Model file for the job. Use its own axes, mm. Face numbers are marked on the shaded views. A direction names the side the tool comes from. Give positions to 0.01 mm unless a question says otherwise; leave off trailing zeros. Loops run counter-clockwise (first coordinate to the right, second up) from the corner with the lowest first, then second, coordinate; pieces in that order, holes last. Notation, with made-up numbers: M -3,25 L 52,25 A26 cw 52,39 Z; hole C 27,-28.75 d2. An arc over 180 degrees is marked long. Answer in a Markdown table with one row per item.
```python
from build123d import *

# Parameters (mm, degrees)
SKETCH1_R                = 5
BOSS_EXTRUDE2_DEPTH      = 26
SKETCH9_R                = 11.5
CUT_EXTRUDE7_DEPTH       = 26
CUT_EXTRUDE8_DEPTH       = 57
BOSS_EXTRUDE5_DEPTH      = 35
BOSS_EXTRUDE5_DEPTH_BACK = 10


with BuildPart() as part:
    # Sketch1 → Boss-Extrude2 (new body)
    with BuildSketch(Plane.XY):
        with BuildLine():
            Line((-13.871543988, -187.456565175), (-0.750718318, -9.931237526))
            Line((-0.750718318, -9.931237526), (-9.971378105, 32.063387678))
            Line((-9.971378105, 32.063387678), (-9.97665526, 32.075234554))
            Line((-9.97665526, 32.075234554), (-9.977087782, 32.075348974))
            Line((-9.977087782, 32.075348974), (-9.978230603, 32.075651298))
            Line((-9.978230603, 32.075651298), (-9.977087779, 32.075655544))
            ThreePointArc((-9.977087779, 32.075655544), (-24.981119404, 47.075655002), (-39.977085612, 32.067592296))
            Line((-39.977085612, 32.067592296), (-40.143970803, 31.267359869))
            Line((-40.143970803, 31.267359869), (-33.520138903, -191.065133081))
            ThreePointArc((-33.520138903, -191.065133081), (-31.855635546, -197.51068285), (-27.565830072, -202.601188939))
            Line((-27.565830072, -202.601188939), (-6.826859709, -218.262215052))
            Line((-6.826859709, -218.262215052), (-2.296825809, -203.937706242))
            Line((-2.296825809, -203.937706242), (-10.96981355, -195.264718501))
            ThreePointArc((-10.96981355, -195.264718501), (-13.272387355, -191.677160819), (-13.871543988, -187.456565175))
        make_face()
        with Locations((-18.750718318, -9.924344456)):
            Circle(SKETCH1_R, mode=Mode.SUBTRACT)
    extrude(amount=BOSS_EXTRUDE2_DEPTH)

    # Sketch9 → Cut-Extrude7 (cut)
    with BuildSketch(Plane.XY):
        with Locations((-24.977087779, 32.075655544)):
            Circle(SKETCH9_R)
    extrude(amount=CUT_EXTRUDE7_DEPTH, mode=Mode.SUBTRACT)

    # Sketch10 → Cut-Extrude8 (cut)
    with BuildSketch(Plane.XY):
        with BuildLine():
            Line((-29.654511548, -21.002260091), (-10.602832717, -21.002260091))
            ThreePointArc((-10.602832717, -21.002260091), (-6.952180176, -22.585721488), (-5.613794584, -26.333165681))
            Line((-5.613794584, -26.333165681), (-9.366001824, -82.90490561))
            ThreePointArc((-9.366001824, -82.90490561), (-10.938501354, -86.224652561), (-14.355039957, -87.574000019))
            Line((-14.355039957, -87.574000019), (-27.922723591, -87.574000019))
            ThreePointArc((-27.922723591, -87.574000019), (-31.403747307, -86.163216354), (-32.920382463, -82.726989577))
            Line((-32.920382463, -82.726989577), (-34.65217042, -26.155249648))
            ThreePointArc((-34.65217042, -26.155249648), (-33.243727882, -22.521236375), (-29.654511548, -21.002260091))
        make_face()
        with BuildLine():
            Line((-14.784895538, -91.270958439), (-27.832276958, -91.270958439))
            ThreePointArc((-27.832276958, -91.270958439), (-31.398552804, -92.766436134), (-32.831514258, -96.358287804))
            Line((-32.831514258, -96.358287804), (-31.399590979, -178.329847134))
            ThreePointArc((-31.399590979, -178.329847134), (-29.904875984, -181.808793615), (-26.400353679, -183.242517768))
            Line((-26.400353679, -183.242517768), (-21.386933453, -183.242517768))
            ThreePointArc((-21.386933453, -183.242517768), (-17.996285711, -181.917229715), (-16.403071948, -178.643920925))
            Line((-16.403071948, -178.643920925), (-9.801034032, -96.672361595))
            ThreePointArc((-9.801034032, -96.672361595), (-11.110183591, -92.880310697), (-14.784895538, -91.270958439))
        make_face()
    extrude(amount=CUT_EXTRUDE8_DEPTH, mode=Mode.SUBTRACT)

    # Sketch11 → Boss-Extrude5 (add, two sides)
    with BuildSketch(Plane.XY) as boss_extrude5_sk:
        with BuildLine():
            Line((-2.296825809, -203.937706242), (-6.826859709, -218.262215052))
            Line((-6.826859709, -218.262215052), (-10.445160296, -229.703714118))
            Line((-10.445160296, -229.703714118), (-8.916301823, -230.367275492))
            ThreePointArc((-8.916301823, -230.367275492), (-6.475373676, -230.344079521), (-4.859724836, -228.514230593))
            Line((-4.859724836, -228.514230593), (3.138639896, -203.047724737))
            ThreePointArc((3.138639896, -203.047724737), (3.748708228, -200.0920804), (3.754779808, -197.074137401))
            Line((3.754779808, -197.074137401), (3.121631235, -190.683812553))
            ThreePointArc((3.121631235, -190.683812553), (2.049929764, -188.669228662), (-0.128962116, -187.991347795))
            Line((-0.128962116, -187.991347795), (-2.151569065, -188.170856397))
            Line((-2.151569065, -188.170856397), (-1.355950129, -197.135465185))
            ThreePointArc((-1.355950129, -197.135465185), (-1.386055005, -200.091588206), (-1.995347326, -202.984395233))
            Line((-1.995347326, -202.984395233), (-2.296825809, -203.937706242))
        make_face()
    extrude(amount=BOSS_EXTRUDE5_DEPTH)
    extrude(boss_extrude5_sk.sketch, amount=-BOSS_EXTRUDE5_DEPTH_BACK)


solid = part.part
```
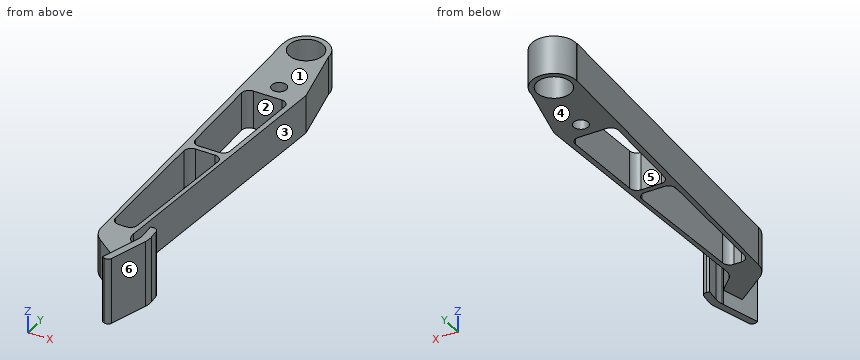
(1) Flat gauge pins, fed straight in: P1, Ø1.5, axis at x = -15, y = -193, coming from the +Z side; P2, Ø16, axis at x = -18.75, y = -9.92, coming from the -Z side; P3, Ø10, axis at x = -22, z = 25.5, coming from the -Y side. Where does each tip first touch, or does it go through?
Established:
| item | result |
|---|---|
| P1 | stops at z = 26 |
| P2 | stops at z = 0 |
| P3 | stops at y = -210.58 |
(2) Mould opens along Y. For the marked faces 4, 5 and 6 say: pulls with the +Y half, pulls with the -Y half, needs draft (parallel to the pull), parting line crosses it, or undercut.
Established:
| item | result |
|---|---|
| face 4 | needs draft |
| face 5 | undercut |
| face 6 | pulls with the -Y half |
(3) Wall check: L1, parallel to Y at x = -24.5, z = 5; L2, parallel to Y at x = -23, z = 12.5; L3, parallel to Y at x = -30.5, z = 13. Give the ranges that are in metal, low to high.
Established:
| item | result |
|---|---|
| L1 | y = -204.92 to -183.24, -91.27 to -87.57, -21 to 20.59, 43.57 to 47.07 |
| L2 | y = -206.05 to -183.24, -91.27 to -87.57, -21 to -12.56, -7.29 to 20.75, 43.4 to 46.94 |
| L3 | y = -199.67 to -181.1, -92.04 to -86.86, -21.07 to 21.99, 42.16 to 46.02 |
(4) Saw through at A-A, the plane y = -160. Give the cut face in (x, z), and give its area (3 significant figures).
Established:
| item | result |
|---|---|
| outline | M -34.45,0 L -31.72,0 L -31.72,26 L -34.45,26 Z; M -14.9,0 L -11.84,0 L -11.84,26 L -14.9,26 Z |
| area | 150 mm2 |
(5) Saw through at B-B, the plane z = 29. Give the cut face in (x, y), and give its area (3 significant figures).
Established:
| item | result |
|---|---|
| outline | M -10.45,-229.7 L -8.92,-230.37 A3 ccw -4.86,-228.51 L 3.14,-203.05 A15 ccw 3.75,-197.07 L 3.12,-190.68 A3 ccw -0.13,-187.99 L -2.15,-188.17 L -1.36,-197.14 A15 cw -2,-202.98 Z |
| area | 216 mm2 |
(6) Saw through at D-D, the plane y = -214. Give the cut face in (x, z), and give its area (3 significant figures).
Established:
| item | result |
|---|---|
| outline | M -12.47,0 L -5.48,0 L -5.48,-10 L -0.3,-10 L -0.3,35 L -5.48,35 L -5.48,26 L -12.47,26 Z |
| area | 415 mm2 |
(7) Saw through at C-C, the plane y = -103. Give the cut face in (x, z).
Established:
| item | result |
|---|---|
| outline | M -36.14,0 L -32.72,0 L -32.72,26 L -36.14,26 Z; M -10.31,0 L -7.63,0 L -7.63,26 L -10.31,26 Z |
(8) Which spindle directions (+Z, -Z, +X, -X, +Y, -Y) get a long thin tool onto all of the face, cutting with end or side? Do the marked faces 1, 2 and 3. Say none if no direction does.
Established:
| item | result |
|---|---|
| face 1 | +Z, -X, +Y |
| face 2 | +Z, -Z |
| face 3 | +Z, -Z, +X |
